from build123d import *

# Parameters (mm, degrees)
SKETCH1_W                      = 33
SKETCH1_H                      = 11
SKETCH1_W_2                    = 30
SKETCH1_H_2                    = 8
BOSS_EXTRUDE1_DEPTH            = 8
SKETCH3_R                      = 0.8
CUT_EXTRUDE3_DEPTH             = 22.38340478
CUT_EXTRUDE5_REACH             = 21.144
SKETCH5_R                      = 3.425
CUT_EXTRUDE5_DIRECTION_2_DEPTH = 20.144189719
CUT_EXTRUDE4_DEPTH             = 22.38340478
CUT_EXTRUDE9_START             = -1.5
CUT_EXTRUDE9_DEPTH             = 8
SKETCH9_W                      = 22
SKETCH9_H                      = 8
CUT_EXTRUDE8_DEPTH             = 2.25
BOSS_EXTRUDE8_START            = 2
SKETCH12_W                     = 28.108309096
SKETCH12_H                     = 11
SKETCH12_R                     = 3.425
BOSS_EXTRUDE8_DEPTH            = 2
FILLET1_R                      = 1
CHAMFER1_SIZE                  = 1.5
CHAMFER1_SIZE_2                = 3.369055161
CHAMFER2_SIZE                  = 0.5
CHAMFER2_SIZE2                 = 1.123018387
CHAMFER3_SIZE                  = 0.5
CHAMFER3_SIZE2                 = 1.123018387


with BuildPart() as part:
    # Sketch1 → Boss-Extrude1 (new body)
    # profile 1 of 2: a face of its own
    with BuildSketch(Plane(origin=(0, 0, 0), x_dir=(1, 0, 0), z_dir=(0, 1, 0))):
        Rectangle(SKETCH1_W, SKETCH1_H)
        Rectangle(SKETCH1_W_2, SKETCH1_H_2, mode=Mode.SUBTRACT)
    # profile 2 of 2: a face of its own
    with BuildSketch(Plane(origin=(0, 0, 0), x_dir=(1, 0, 0), z_dir=(0, 1, 0))):
        Rectangle(SKETCH1_W_2, SKETCH1_H_2)
    extrude(amount=BOSS_EXTRUDE1_DEPTH)

    # Sketch3 → Cut-Extrude3 (cut, through all)
    with BuildSketch(Plane.XY.offset(5.5)):
        with Locations((-12.5, 4)):
            Circle(SKETCH3_R)
        with Locations((12.5, 4)):
            Circle(SKETCH3_R)
    extrude(amount=-CUT_EXTRUDE3_DEPTH, mode=Mode.SUBTRACT)

    # Sketch5 → Cut-Extrude5 (cut, up to next)
    with BuildSketch(Plane(origin=(0, 8, 0), x_dir=(1, 0, 0), z_dir=(0, 1, 0)), mode=Mode.PRIVATE) as cut_extrude5_sk1:
        with Locations(Location((0, 0, 0), (0, 0, 90))):
            Circle(SKETCH5_R)
    cut_extrude5_tool1 = extrude(cut_extrude5_sk1.sketch, amount=-CUT_EXTRUDE5_REACH, mode=Mode.PRIVATE) & part.part
    add(cut_extrude5_tool1.solids().sort_by_distance((0, 8, 0))[0], mode=Mode.SUBTRACT)

    # Sketch5 → Cut-Extrude5 direction 2 (cut)
    with BuildSketch(Plane(origin=(0, 8, 0), x_dir=(1, 0, 0), z_dir=(0, 1, 0))):
        with Locations(Location((0, 0, 0), (0, 0, 90))):
            Circle(SKETCH5_R)
    extrude(amount=CUT_EXTRUDE5_DIRECTION_2_DEPTH, mode=Mode.SUBTRACT)

    # Sketch4 → Cut-Extrude4 (cut, through all)
    with BuildSketch(Plane.XY.offset(5.5)):
        Polygon((-16.5, 0), (-14.054154548, 8), (-16.5, 8), align=None)
        Polygon((16.5, 0), (14.054154548, 8), (16.5, 8), align=None)
    extrude(amount=-CUT_EXTRUDE4_DEPTH, mode=Mode.SUBTRACT)

    # Sketch14 → Cut-Extrude9 (cut)
    with BuildSketch(Plane.XY.offset(5.5).offset(CUT_EXTRUDE9_START)):
        Polygon((-15, 0), (15, 0), (14.235673296, 2.5), (-14.235673296, 2.5), align=None)
    extrude(amount=-CUT_EXTRUDE9_DEPTH, mode=Mode.SUBTRACT)

    # Sketch9 → Cut-Extrude8 (cut)
    with BuildSketch(Plane.XZ.offset(-2.5)):
        Rectangle(SKETCH9_W, SKETCH9_H)
    extrude(amount=-CUT_EXTRUDE8_DEPTH, mode=Mode.SUBTRACT)

    # Sketch12 → Boss-Extrude8 (add)
    with BuildSketch(Plane(origin=(0, 8, 0), x_dir=(1, 0, 0), z_dir=(0, 1, 0)).offset(BOSS_EXTRUDE8_START)):
        Rectangle(SKETCH12_W, SKETCH12_H)
        with Locations(Location((0, 0, 0), (0, 0, 90))):
            Circle(SKETCH12_R, mode=Mode.SUBTRACT)
    extrude(amount=-BOSS_EXTRUDE8_DEPTH)

    # Fillet1
    fillet1_edges = [part.edges().sort_by_distance(p)[0] for p in [
        (0, 10, 5.5),
        (0, 10, -5.5),
    ]]
    fillet(fillet1_edges, radius=FILLET1_R)

    # Chamfer1
    # the kernel refuses this chamfer: 3.369055161, 1.5 mm, written as the material it takes off along each edge
    with BuildSketch(Plane(origin=(0, 4.75, 0), x_dir=(0, 0, -1), z_dir=(1, 0, 0))) as chamfer1_piece_1_section:
        Polygon((3.425, CHAMFER1_SIZE), (3.425 + CHAMFER1_SIZE_2, 0), (3.425, 0), align=None)
    chamfer1_piece_1 = revolve(axis=Axis((0, 4.75, 0), (0, 1, 0)), mode=Mode.PRIVATE)
    chamfer1_piece_1 = split(chamfer1_piece_1, bisect_by=Plane(origin=(-3.367570152, 6.000830153, 4), z_dir=(0, 0, -1)), keep=Keep.TOP, mode=Mode.PRIVATE)
    chamfer1_piece_1 = split(chamfer1_piece_1, bisect_by=Plane(origin=(-3.367570152, 6.000830153, -4), z_dir=(0, 0, 1)), keep=Keep.TOP, mode=Mode.PRIVATE)
    add(chamfer1_piece_1, mode=Mode.SUBTRACT)

    # Chamfer2
    chamfer2_edges = [part.edges().sort_by_distance(p)[0] for p in [
        (-11, 2.5, 0),
    ]]
    chamfer2_side = [part.faces().sort_by_distance(p)[0] for p in [
        (-11, 3.625, 0),
    ]]
    chamfer(chamfer2_edges, length=CHAMFER2_SIZE, length2=CHAMFER2_SIZE2, reference=chamfer2_side[0])

    # Chamfer3
    chamfer3_edges = [part.edges().sort_by_distance(p)[0] for p in [
        (11, 2.5, 0),
    ]]
    chamfer3_side = [part.faces().sort_by_distance(p)[0] for p in [
        (11, 3.625, 0),
    ]]
    chamfer(chamfer3_edges, length=CHAMFER3_SIZE, length2=CHAMFER3_SIZE2, reference=chamfer3_side[0])


solid = part.part
Here's how the part is built. I have some questions about the finished solid (model axes, mm). A direction names the side the tool comes from. Coordinates: 2 decimals unless noted, no trailing zeros. Order: outer loops, then holes, each group sorted by start corner. A loop starts at its lowest first (then second) coordinate and runs counter-clockwise, first axis right, second up. Notation, with made-up numbers: M -35,56.5 L 20,56.5 A15 ccw 20,81.5 Z; hole C 25.5,-7 d6. An arc over 180 degrees is marked long. Answer as CSV lines item,"result". Start each with the question number.
1. I want a section at D-D, the plane x = -8. Write out the boundary of the cut face in (y, z).
2. I want a section at C-C, the plane y = 4. Write out the boundary of the cut face in (x, z).
3. On a 3-axis mill with a long thin cutter (end or side, diameter ignored), from which of +Z, -Z, +X, -X, +Y, -Y can I reach the whole of each face in a straight line? I mean faces 1 (the flat face through (14.054, 9, 0)), 2 (the flat face through (-14.054, 9, 0)), 3 (the flat face through (0, 2, 4)), 4 (the flat face through (0, 5, -5.5)), 5 (the cylindrical face through (-1.029, 8.151, -3.267)). Say none if no direction works.
4. I need wall thicknesses on line 1 (Z direction, x = 0, y = 7.5) (3 decimals); line 2 (Z direction, x = -6, y = 3); line 3 (Y direction, x = 12.5, z = -1.75). Which ranges of each line are inside material? Lowest first, please. Write a range as [from, to].
5. We'd pull the mould along Y, two halves only. Please class faces 6 (the flat face through (0, 5, 5.5)), 7 (the flat face through (9, 4.75, 0)), 8 (the cylindrical face through (-13.13, 3.51, 0.08)): released by +Y, released by -Y, zero draft, split by the parting line, or undercut.
6. I want a section at A-A, the plane z = 0. Write out the boundary of the cut face in (x, y) (3 decimals), and give its area (3 significant figures).
7. For pin 1 (0.6 mm diameter, centred on x = 13.5, z = 0.5, fed in from -Y); pin 2 (0.9 mm diameter, centred on y = 4, z = 0, fed in from -X); pin 3 (1 mm diameter, centred on y = 9, z = -1.5, fed in from +X); pin 4 (2 mm diameter, centred on x = -12.5, y = 4, fed in from -Z), each with a flat end and sliding along its axis, tell me the tip position at first contact or that it passes through.
8. I want a section at B-B, the plane x = 12.5. Write out the boundary of the cut face in (y, z), and give its area (3 significant figures).
Recorded:
1,outline,"M 0,-5.5 L 9,-5.5 A1 ccw 10,-4.5 L 10,4.5 A1 ccw 9,5.5 L 0,5.5 L 0,4 L 4.75,4 L 4.75,-4 L 0,-4 Z"
2,outline,"M -15.28,-5.5 L -13.3,-5.5 L -13.3,5.5 L -15.28,5.5 Z; M -11.7,-5.5 L 11.7,-5.5 L 11.7,5.5 L -11.7,5.5 Z; M 13.3,-5.5 L 15.28,-5.5 L 15.28,5.5 L 13.3,5.5 Z; hole M -11,-4 L 11,-4 L 11,4 L -11,4 Z"
3,face 1,"+Z, -Z, +X, +Y"
3,face 2,"+Z, -Z, -X, +Y"
3,face 3,"-Y"
3,face 4,"-Z, +X, -X, +Y, -Y"
3,face 5,"+Y, -Y"
4,line 1,"z = [-5.5, -3.425], [3.425, 5.5]"
4,line 2,"z = [-5.5, -4], [4, 5.5]"
4,line 3,"y = [2.5, 3.2], [4.8, 10]"
5,face 6,"zero draft"
5,face 7,"released by -Y"
5,face 8,"undercut"
6,outline,"M -16.5,0 L -15,0 L -14.236,2.5 L -12.123,2.5 L -11,3 L -11,4.75 L -6.794,4.75 L -3.425,6.25 L -3.425,10 L -14.054,10 L -14.054,8 Z; M 3.425,6.25 L 6.794,4.75 L 11,4.75 L 11,3 L 12.123,2.5 L 14.236,2.5 L 15,0 L 16.5,0 L 14.054,8 L 14.054,10 L 3.425,10 Z; hole C -12.5,4 d1.6; hole C 12.5,4 d1.6"
6,area,"132 mm2"
7,pin 1,"stops at y = 2.5"
7,pin 2,"stops at x = -15.41"
7,pin 3,"stops at x = 14.05"
7,pin 4,"stops at z = -5.5"
8,outline,"M 0,-5.5 L 3.2,-5.5 L 3.2,5.5 L 0,5.5 L 0,4 L 2.5,4 L 2.5,-4 L 0,-4 Z; M 4.8,-5.5 L 9,-5.5 A1 ccw 10,-4.5 L 10,4.5 A1 ccw 9,5.5 L 4.8,5.5 Z"
8,area,"72.0 mm2"
